from build123d import *

# Parameters (mm, degrees)
SKETCH1_R           = 25
BOSS_EXTRUDE1_DEPTH = 6
SKETCH2_W           = 20
SKETCH2_H           = 20
BOSS_EXTRUDE2_DEPTH = 30
BOSS_EXTRUDE3_DEPTH = 20
FILLET1_R           = 10
FILLET2_R           = 10
SKETCH4_R           = 11.1
CUT_EXTRUDE1_DEPTH  = 2.2
SKETCH5_R           = 1.65
CUT_EXTRUDE2_DEPTH  = 80


with BuildPart() as part:
    # Sketch1 → Boss-Extrude1 (new body)
    with BuildSketch(Plane(origin=(0, 0, 0), x_dir=(1, 0, 0), z_dir=(0, 1, 0))):
        with Locations(Location((0, 0, 0), (0, 0, 270))):
            Circle(SKETCH1_R)
    extrude(amount=BOSS_EXTRUDE1_DEPTH)

    # Sketch2 → Boss-Extrude2 (add)
    with BuildSketch(Plane(origin=(0, 6, 0), x_dir=(1, 0, 0), z_dir=(0, 1, 0))):
        Rectangle(SKETCH2_W, SKETCH2_H)
    extrude(amount=BOSS_EXTRUDE2_DEPTH)

    # Sketch3 → Boss-Extrude3 (add)
    with BuildSketch(Plane.ZY.offset(10)):
        Polygon((-10, 36), (-31.5, 52.965778424), (-31.5, 102.965778424), (-21.5, 102.965778424), (-21.5, 58.01124712), (21.5, 58.01124712), (21.5, 102.965778424), (31.5, 102.965778424), (31.5, 52.965778424), (10, 36), align=None)
    extrude(amount=-BOSS_EXTRUDE3_DEPTH)

    # Fillet1
    fillet1_edges = [part.edges().sort_by_distance(p)[0] for p in [
        (0, 58.01124712, -21.5),
    ]]
    fillet(fillet1_edges, radius=FILLET1_R)

    # Fillet2
    fillet2_edges = [part.edges().sort_by_distance(p)[0] for p in [
        (0, 58.01124712, 21.5),
    ]]
    fillet(fillet2_edges, radius=FILLET2_R)

    # Sketch4 → Cut-Extrude1 (cut)
    with BuildSketch(Plane.XZ):
        with Locations(Location((0, 0, 0), (0, 0, 270))):
            Circle(SKETCH4_R)
    extrude(amount=-CUT_EXTRUDE1_DEPTH, mode=Mode.SUBTRACT)

    # Sketch5 → Cut-Extrude2 (cut)
    with BuildSketch(Plane.XY.offset(31.5)):
        with Locations((4.734939198, 89.684875187)):
            Circle(SKETCH5_R)
        with Locations((-2.682610937, 97.102425322)):
            Circle(SKETCH5_R)
        with Locations((-5.122436395, 93.272666491)):
            Circle(SKETCH5_R)
    extrude(amount=-CUT_EXTRUDE2_DEPTH, mode=Mode.SUBTRACT)


solid = part.part
Source: CAD feature listing. Evaluate the final solid. Frame: model axes, mm. A direction names the side the tool comes from. Give positions to 0.01 mm unless a question says otherwise; leave off trailing zeros. Write each loop counter-clockwise with the first axis right and the second up, starting at its lowest first coordinate (ties: lowest second). Pieces come first, ordered by that corner, then holes. Notation, with made-up numbers: (-15, 82) - (16, 82) arc R25 cw to (16, 108) - close; hole circle Ø9 at (82.5, 2). An arc over 180 degrees is marked (long way). Write item = value, one per line. Start each with the question number.
Q1. Cut plane D-D, the plane z = 13.5. Return loops of the section in (x, y), then the cut area to 3 significant figures.
Q2. Cut plane B-B, the plane z = -27. Return loops of the section in (x, y), then the cut area to 3 significant figures.
Q3. Pin query (flat end, axial travel): pin 1 Ø4 at (y, z) = (34.5, 10.5) entering from +X; pin 2 Ø6 at (x, z) = (4, 4.5) entering from +Y; pin 3 Ø8 at (x, z) = (17, 1) entering from +Y. Return the tip coordinate at first contact, or that it passes through.
Q4. Material intervals for probe 1 along Z at (x, y) = (-8.5, 85); probe 2 along Y at (x, z) = (11.5, 6); probe 3 along X at (y, z) = (36, 1), sorted ascending.
Q5. Cut plane C-C, the plane y = 16. Return loops of the section in (x, z).
Q6. Draft query along Y for faces 1 (the flat face through (0, 85, 21.5)), 2 (the cylindrical face through (0.14, 60.86, 18.49)), 3 (the cylindrical face through (-3.04, 95.49, -26.43)). Return one class per face: +Y half, -Y half, draft (parallel to the pull), parting line (faces both ways), or undercut.
Q7. Cut plane A-A, the plane z = 0. Return loops of the section in (x, y), then the cut area to 3 significant figures.
Q8. Reachability of faces 4 (the flat face through (0, 58.011, 0)), 5 (the flat face through (-0.14, 44.364, -20.6)), 6 (the flat face through (-0.1, 44.6, 20.9)), 7 (the flat face through (10, 55, 0)) from +Z, -Z, +X, -X, +Y, -Y: full face, straight path, thin tool, end or side. Return the list, or none.
Computed values:
q1.outline = (-21.04, 0) - (21.04, 0) - (21.04, 6) - (-21.04, 6) - close; (-10, 38.76) - (10, 38.76) - (10, 58.21) - (-10, 58.21) - close
q1.area = 642 mm²
q2.outline = (-10, 49.41) - (10, 49.41) - (10, 102.97) - (-10, 102.97) - close; hole circle Ø3.3 at (-5.12, 93.27); hole circle Ø3.3 at (-2.68, 97.1); hole circle Ø3.3 at (4.73, 89.68)
q2.area = 1,050 mm²
q3.pin_1 = 10
q3.pin_2 = 58.01
q3.pin_3 = 6
q4.probe_1 = -31.5 to -21.5, 21.5 to 31.5
q4.probe_2 = 0 to 6
q4.probe_3 = -10 to 10
q5.outline = (-10, -10) - (10, -10) - (10, 10) - (-10, 10) - close
q6.face_1 = draft
q6.face_2 = +Y half
q6.face_3 = undercut
q7.outline = (-25, 0) - (-11.1, 0) - (-11.1, 2.2) - (11.1, 2.2) - (11.1, 0) - (25, 0) - (25, 6) - (10, 6) - (10, 58.01) - (-10, 58.01) - (-10, 6) - (-25, 6) - close
q7.area = 1,290 mm²
q8.face_4 = +X, -X, +Y
q8.face_5 = -Z, +X, -X
q8.face_6 = +Z, +X, -X
q8.face_7 = +Z, -Z, +X, +Y
